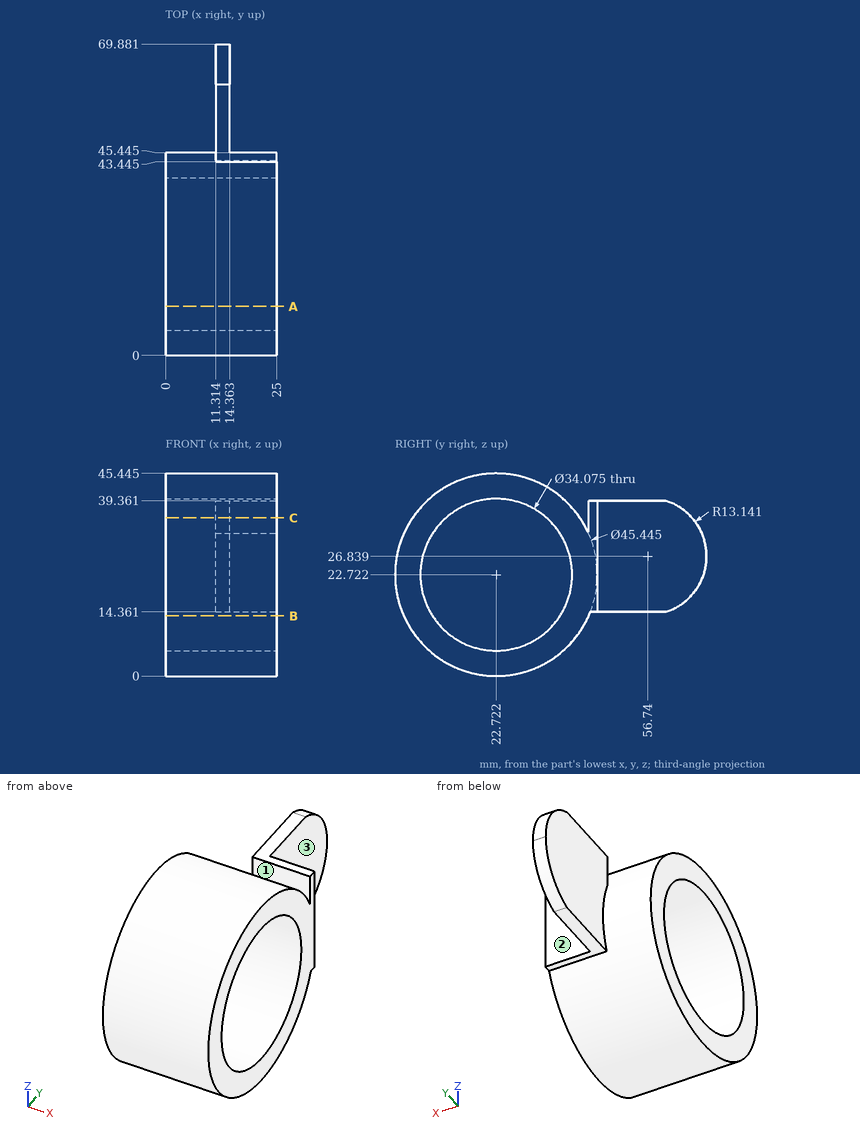
Source: three-view drawing plus pictorial views. Frame: mm from the lowest corner of the part. Round coordinates to 2 decimals unless told otherwise and drop trailing zeros. Write each loop counter-clockwise with the first axis right and the second up, starting at its lowest first coordinate (ties: lowest second). Pieces come first, ordered by that corner, then holes. Notation, with made-up numbers: M -17.75,89.5 L 3.25,89.5 A10 ccw 3.25,98.5 Z; hole C 74,-16 d5. An arc over 180 degrees is marked long. Use CSV: the item, a comma, the result in double quotes. Start each with the question number.
Q1. Cut plane A-A on y = 11. Output: boundary loops of the cut face in (x, z), plus the area to 3 significant figures.
Q2. Cut plane B-B on z = 13.5. Output: boundary loops of the cut face in (x, y) (1 decimal).
Q3. Pull-direction query (Y, two-part tool) for the marked faces 1, 2 and 3; classes: +Y half, -Y half, draft (parallel to the pull), parting line (faces both ways), or undercut.
Q4. Cut plane C-C on z = 35.5. Output: boundary loops of the cut face in (x, y) (1 decimal).
Q5. Line query: line 1 (Y direction, x = 17, z = 35) (1 decimal); line 2 (Y direction, x = 3, z = 22) (1 decimal). Output: solid intervals per line, ascending. Write a range as from..to.
Q6. First-contact query: P1, Ø2, axis at x = 12.5, z = 31.5, coming from the -Y side; P2, Ø1.5, axis at x = 9, y = 13.5, coming from the +Z side; P3, Ø4, axis at x = 16, y = 50.5, coming from the -Z side; P4, Ø11, axis at x = 20.5, y = 53.5, coming from the +Z side. Flat tips, straight axial feed; report the tip coordinate or a pass-through.
Results found:
1,outline,"M 0,3.26 L 25,3.26 L 25,10.36 L 0,10.36 Z; M 0,35.09 L 25,35.09 L 25,42.19 L 0,42.19 Z"
1,area,"355 mm^2"
2,outline,"M 0,2 L 25,2 L 25,8.4 L 0,8.4 Z; M 0,37 L 25,37 L 25,43.5 L 0,43.5 Z"
3,face 1,"undercut"
3,face 2,"+Y half"
3,face 3,"draft"
4,outline,"M 0,3.9 L 25,3.9 L 25,11.5 L 0,11.5 Z; M 0,34 L 25,34 L 25,41.5 L 0,41.5 Z; M 11.3,43.4 L 25,43.4 L 25,45.4 L 14.4,45.4 L 14.4,66.6 L 11.3,66.6 Z"
5,line 1,"3.6..10.9, 34.5..41.8, 43.4..45.4"
5,line 2,"0..5.7, 39.7..45.4"
6,P1,"y = 1.37"
6,P2,"z = 43.81"
6,P3,"z = 14.36"
6,P4,"through"
